Could you check a few things on this model? Use its own coordinates, in mm. Give positions to 0.01 mm unless a question says otherwise; leave off trailing zeros. Loops run counter-clockwise (first coordinate to the right, second up) from the corner with the lowest first, then second, coordinate; pieces in that order, holes last. Notation, with made-up numbers: (40.25, 60.5) - (94.25, 60.5) arc R24 cw to (94.25, 80.5) - close; hole circle Ø8 at (18, 61). An arc over 180 degrees is marked (long way). Answer in a Markdown table with one row per item. Add a question column.
```python
from build123d import *

# Parameters (mm, degrees)
SKETCH1_W           = 114.3
SKETCH1_H           = 114.3
SKETCH1_R           = 50.8
SKETCH1_R_2         = 2.032
BOSS_EXTRUDE1_DEPTH = 3
SKETCH3_W           = 50
SKETCH3_H           = 3
BOSS_EXTRUDE2_DEPTH = 35.56
SKETCH4_R           = 8
CUT_EXTRUDE1_DEPTH  = 4
FILLET2_R           = 8.89


with BuildPart() as part:
    # Sketch1 → Boss-Extrude1 (new body)
    with BuildSketch(Plane(origin=(0, 0, 0), x_dir=(1, 0, 0), z_dir=(0, 1, 0))):
        with Locations((57.15, 57.15)):
            Rectangle(SKETCH1_W, SKETCH1_H)
        with Locations((57.15, 57.15)):
            Circle(SKETCH1_R, mode=Mode.SUBTRACT)
        with Locations((11.43, 102.87)):
            Circle(SKETCH1_R_2, mode=Mode.SUBTRACT)
        with Locations((102.87, 102.87)):
            Circle(SKETCH1_R_2, mode=Mode.SUBTRACT)
        with Locations((102.87, 11.43)):
            Circle(SKETCH1_R_2, mode=Mode.SUBTRACT)
        with Locations((11.43, 11.43)):
            Circle(SKETCH1_R_2, mode=Mode.SUBTRACT)
    boss_extrude1 = extrude(amount=BOSS_EXTRUDE1_DEPTH)

    # Mirror1: Boss-Extrude1 across plane
    add(boss_extrude1.mirror(Plane(origin=(114.3, 3, 0), x_dir=(0, 0, 1), z_dir=(-1, 0, 0))))

    # Sketch3 → Boss-Extrude2 (add)
    with BuildSketch(Plane.XY):
        with Locations((114.3, 1.5)):
            Rectangle(SKETCH3_W, SKETCH3_H)
    extrude(amount=BOSS_EXTRUDE2_DEPTH)

    # Sketch4 → Cut-Extrude1 (cut, through all)
    with BuildSketch(Plane(origin=(0, 3, 0), x_dir=(1, 0, 0), z_dir=(0, 1, 0))):
        with Locations((101.3, -24.06)):
            Circle(SKETCH4_R)
        with Locations((127.3, -24.06)):
            Circle(SKETCH4_R)
    extrude(amount=-CUT_EXTRUDE1_DEPTH, mode=Mode.SUBTRACT)

    # Fillet2
    fillet2_edges = [part.edges().sort_by_distance(p)[0] for p in [
        (139.3, 1.5, 0),
        (89.3, 1.5, 0),
        (139.3, 1.5, 35.56),
        (89.3, 1.5, 35.56),
    ]]
    fillet(fillet2_edges, radius=FILLET2_R)


solid = part.part
```
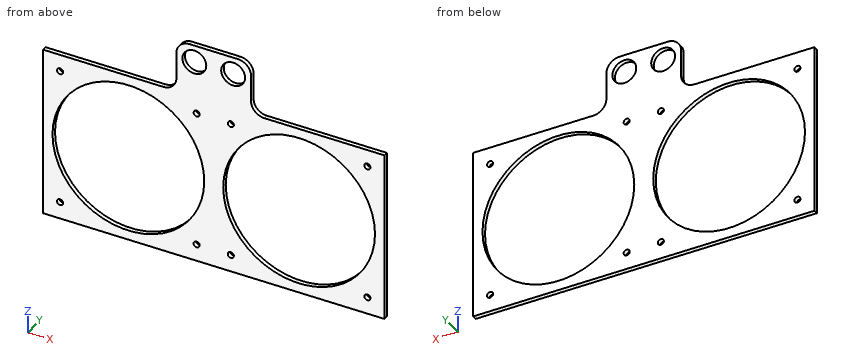
(1) I want a section at A-A on x = 57.15. Please give me the cut outline in (y, z), then the cut area to 3 significant figures.
(2) I want a section at B-B on y = 1.6. State how many separate pieces and enclosed holes the cut face has, then the cut area to 3 significant figures.
(3) I want a section at C-C on z = -98.5. Please give me the cut outline in (x, y), then the cut area to 3 significant figures.
(4) Please list where these lines run through material, in increasing order: line 1 (X direction, y = 1.9, z = 24.06); line 2 (X direction, y = 2.45, z = -59); line 3 (Z direction, x = 217.17, y = 0.85).
(5) For pin 1 Ø4.5 at (x, z) = (217.17, -11.43) entering from -Y; pin 2 Ø1.5 at (y, z) = (1.5, 20.5) entering from +X, each with a flat end and sliding along its axis, tell me the tip position at first contact or that it passes through.
(6) I want a section at D-D on x = 176. Please give me the cut outline in (y, z), then the cut area to 3 significant figures.
Reported:
| question | item | result |
|---|---|---|
| 1 | outline | (0, -114.3) - (3, -114.3) - (3, -107.95) - (0, -107.95) - close; (0, -6.35) - (3, -6.35) - (3, 0) - (0, 0) - close |
| 1 | area | 38.1 mm² |
| 2 | separate pieces | 1 |
| 2 | enclosed holes | 12 |
| 2 | area | 11,200 mm² |
| 3 | outline | (0, 0) - (27.64, 0) - (27.64, 3) - (0, 3) - close; (86.66, 0) - (141.94, 0) - (141.94, 3) - (86.66, 3) - close; (200.96, 0) - (228.6, 0) - (228.6, 3) - (200.96, 3) - close |
| 3 | area | 332 mm² |
| 4 | line 1 | 89.3 to 93.3, 109.3 to 119.3, 135.3 to 139.3 |
| 4 | line 2 | 0 to 6.38, 107.92 to 120.68, 222.22 to 228.6 |
| 4 | line 3 | -114.3 to -104.9, -100.84 to -79.29, -35.01 to -13.46, -9.4 to 0 |
| 5 | pin 1 | y = 0 |
| 5 | pin 2 | x = 139.3 |
| 6 | outline | (0, -114.3) - (3, -114.3) - (3, -107.75) - (0, -107.75) - close; (0, -6.55) - (3, -6.55) - (3, 0) - (0, 0) - close |
| 6 | area | 39.3 mm² |
